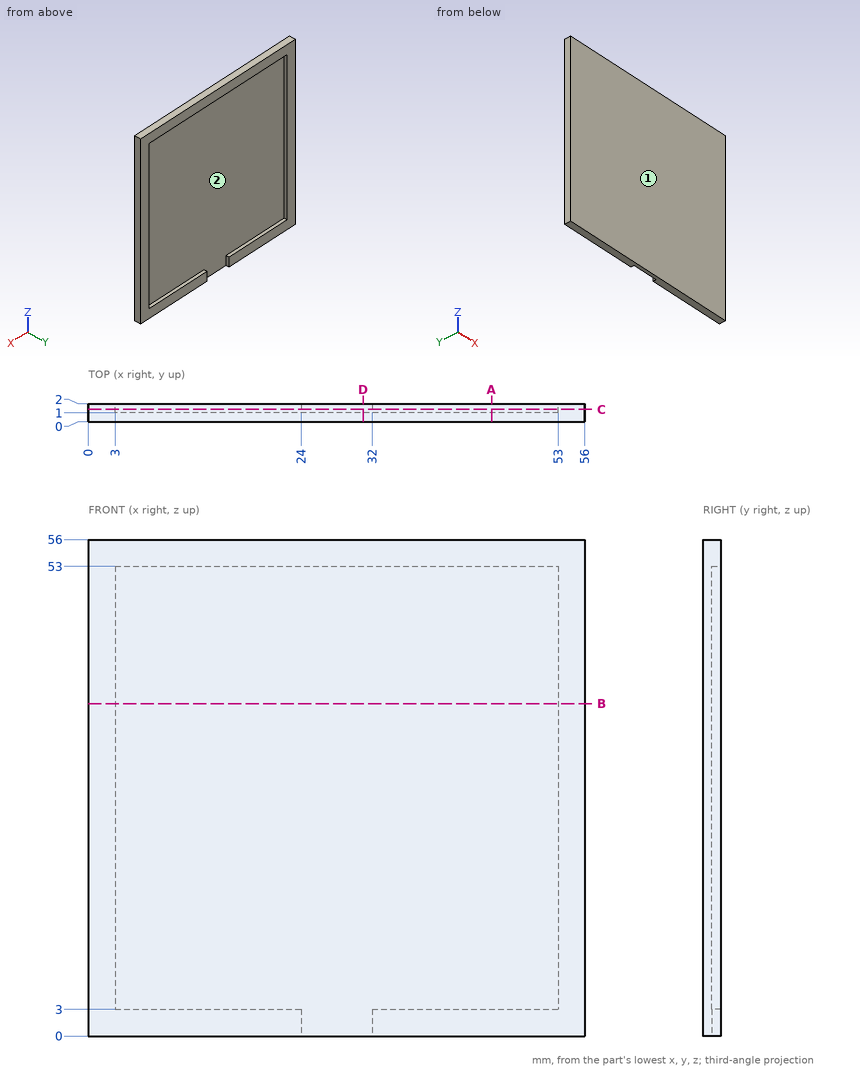
Can you work these out from the drawing? Everything is in mm from the part's minimum corner. Give positions to 0.01 mm unless a question says otherwise; leave off trailing zeros. Order: outer loops, then holes, each group sorted by start corner. A loop starts at its lowest first (then second) coordinate and runs counter-clockwise, first axis right, second up. Notation, with made-up numbers: M 5,39 L 9,39 A19 cw 9,76 Z; hole C 62.25,11.25 d1. An arc over 180 degrees is marked long. Use a Markdown table: item, result. Add a question column.
Item 1: Will this pin go through, and if not, where does the flat tip stop? pin 1 (2 mm diameter, centred on x = 39.5, z = 9, fed in from -Y).
Item 2: Suppose I cut it at B-B (z = 37.5). List the corners of the cut face in (x, y) for me.
Item 3: If I drill on L1, parallel to X at y = 1.4, z = 44; L2, parallel to Y at x = 24.5, z = 32, over which ranges is the centre line in solid material (lowest first)? Write a range as [from, to].
Item 4: Suppose I cut it at D-D (x = 31). List the corners of the cut face in (y, z) for me.
Item 5: Suppose I cut it at C-C (y = 1.4). List the corners of the cut face in (x, z) for me.
Item 6: We'd pull the mould along X, two halves only. Please class the marked faces 1 and 2: +X half, -X half, draft (parallel to the pull), parting line (faces both ways), or undercut.
Item 7: Suppose I cut it at A-A (x = 45.5). List the corners of the cut face in (y, z) for me, then the cut area to 3 significant figures.
Answer sheet:
| question | item | result |
|---|---|---|
| 1 | pin 1 | stops at y = 0 |
| 2 | outline | M 0,0 L 56,0 L 56,2 L 53,2 L 53,1 L 3,1 L 3,2 L 0,2 Z |
| 3 | L1 | x = [0, 3], [53, 56] |
| 3 | L2 | y = [0, 1] |
| 4 | outline | M 0,0 L 1,0 L 1,53 L 2,53 L 2,56 L 0,56 Z |
| 5 | outline | M 0,0 L 24,0 L 24,3 L 3,3 L 3,53 L 53,53 L 53,3 L 32,3 L 32,0 L 56,0 L 56,56 L 0,56 Z |
| 6 | face 1 | draft |
| 6 | face 2 | undercut |
| 7 | outline | M 0,0 L 2,0 L 2,3 L 1,3 L 1,53 L 2,53 L 2,56 L 0,56 Z |
| 7 | area | 62.0 mm² |
